```python
from build123d import *

# Parameters (mm, degrees)
F0_R     = 19.05
F0_R_2   = 17.5
F0_R_3   = 9
F1_DEPTH = 88.9
F2_DEPTH = 13
F3_R     = 17.5
F3_R_2   = 9
F4_DEPTH = 13
F6_W     = 19.05
F6_H     = 15.875
F7_DEPTH = 2.54
F8_D     = 3.7973
F8_DEPTH = 12.7
F8_START = 2.54
F8_TIP   = 1.1408240143


with BuildPart() as f1:
    # F0 (on Top) → F1 (new body)
    with BuildSketch(Plane.XY):
        Circle(F0_R)
        Circle(F0_R_2, mode=Mode.SUBTRACT)
        Circle(F0_R_2)
        Circle(F0_R_3, mode=Mode.SUBTRACT)
    extrude(amount=F1_DEPTH)

    # F0 (on Top) → F2 (cut)
    with BuildSketch(Plane.XY):
        Circle(F0_R_2)
        Circle(F0_R_3, mode=Mode.SUBTRACT)
    extrude(amount=F2_DEPTH, mode=Mode.SUBTRACT)

    # F3 (on face) → F4 (cut)
    with BuildSketch(Plane.XY.offset(88.9)):
        Circle(F3_R)
        Circle(F3_R_2, mode=Mode.SUBTRACT)
    extrude(amount=-F4_DEPTH, mode=Mode.SUBTRACT)

    # F6 (on offset) → F7 (cut)
    with BuildSketch(Plane.XZ.offset(19.05)):
        with Locations((0, 63.5)):
            Rectangle(F6_W, F6_H)
    extrude(amount=-F7_DEPTH, mode=Mode.SUBTRACT)

    # F8
    # its depths count from where the whole tool has entered the part; down to there all is cleared
    with Locations(Plane.XZ.offset(19.05).offset(-F8_START)):
        with Locations((0, 63.5)):
            Hole(F8_D / 2, depth=F8_DEPTH)
            with Locations((0, 0, -(F8_DEPTH + F8_TIP / 2))):  # 118° drill point
                Cone(0, F8_D / 2, F8_TIP, mode=Mode.SUBTRACT)


solid = f1.part
```
Input: part model. Units: mm. Frame: model coordinates. A direction names the side the tool comes from. Give positions to 0.01 mm unless a question says otherwise; leave off trailing zeros. Order: outer loops, then holes, each group sorted by start corner. A loop starts at its lowest first (then second) coordinate and runs counter-clockwise, first axis right, second up. Notation, with made-up numbers: (0, 13) -> (8, 13) arc R7 ccw to (8, 24) -> close; hole circle Ø10 at (-24.75, 44.5). An arc over 180 degrees is marked (long way). Write each question's results on one line, items separated by ' | '. Start each with the question number.
Item 1: Cut plane A-A on x = 0. Return the cut outline in (y, z).
Item 2: Cut plane C-C on y = -13. Return the cut outline in (x, z), then the cut area to 3 significant figures.
Item 3: Cut plane D-D on x = -14. Return the cut outline in (y, z), then the cut area to 3 significant figures.
Item 4: Mould query, pull axis Y, two halves, no side actions, for faces 4 (the cylindrical face through (-2.48, 18.888, 43.828)), 5 (the flat face through (17, -6, 0)), 6 (the cylindrical face through (-1.172, 8.923, 44.01)). Classes: pulls with the +Y half, pulls with the -Y half, needs draft (parallel to the pull), parting line crosses it, or undercut.
Item 5: Set-up query: faces 1 (the flat face through (0, -18, 55.562)), 2 (the cylindrical face through (0.412, -12.597, 61.646)), 3 (the flat face through (8, -8, 75.9)). Return all of +Z, -Z, +X, -X, +Y, -Y with unobstructed straight access to the full face (end or side cutting, diameter ignored); none if empty.
Item 6: Contact query for flat-ended pins moving along their axis: P1, Ø3.5, axis at x = 0, z = 63.5, coming from the -Y side; P2, Ø17.5, axis at x = -8, y = -2, coming from the -Z side; P3, Ø6, axis at x = 4.5, y = -1.5, coming from the +Z side; P4, Ø6, axis at x = -14, z = 68.5, coming from the +Y side. Output: stop coordinate, or through.
Item 7: Line query: line 1 (Y direction, x = 0, z = 85.25); line 2 (Y direction, x = 0, z = 36); line 3 (Z direction, x = 0, y = -13.5). Output: solid intervals per line, ascending.
Item 8: Cut plane B-B on y = 0. Return the cut outline in (x, z).
Established:
1) outline: (-19.05, 0) -> (-17.5, 0) -> (-17.5, 13) -> (-9, 13) -> (-9, 61.6) -> (-16.51, 61.6) -> (-16.51, 55.56) -> (-19.05, 55.56) -> close; (-19.05, 71.44) -> (-16.51, 71.44) -> (-16.51, 65.4) -> (-9, 65.4) -> (-9, 75.9) -> (-17.5, 75.9) -> (-17.5, 88.9) -> (-19.05, 88.9) -> close; (9, 13) -> (17.5, 13) -> (17.5, 0) -> (19.05, 0) -> (19.05, 88.9) -> (17.5, 88.9) -> (17.5, 75.9) -> (9, 75.9) -> close
2) outline: (-13.92, 0) -> (-11.72, 0) -> (-11.72, 13) -> (11.72, 13) -> (11.72, 0) -> (13.92, 0) -> (13.92, 88.9) -> (11.72, 88.9) -> (11.72, 75.9) -> (-11.72, 75.9) -> (-11.72, 88.9) -> (-13.92, 88.9) -> close; hole circle Ø3.8 at (0, 63.5) | area: 1,860 mm^2
3) outline: (-12.92, 0) -> (-10.5, 0) -> (-10.5, 13) -> (10.5, 13) -> (10.5, 0) -> (12.92, 0) -> (12.92, 88.9) -> (10.5, 88.9) -> (10.5, 75.9) -> (-10.5, 75.9) -> (-10.5, 88.9) -> (-12.92, 88.9) -> close | area: 1,750 mm^2
4) face 4: parting line crosses it | face 5: needs draft | face 6: undercut
5) face 1: +X, -X, -Y | face 2: -Y | face 3: +Z
6) P1: y = 8.83 | P2: z = 13 | P3: through | P4: y = 15.55
7) line 1: -19.05 to -17.5, 17.5 to 19.05 | line 2: -19.05 to -9, 9 to 19.05 | line 3: 13 to 61.6, 65.4 to 75.9
8) outline: (-19.05, 0) -> (-17.5, 0) -> (-17.5, 13) -> (-9, 13) -> (-9, 75.9) -> (-17.5, 75.9) -> (-17.5, 88.9) -> (-19.05, 88.9) -> close; (9, 13) -> (17.5, 13) -> (17.5, 0) -> (19.05, 0) -> (19.05, 88.9) -> (17.5, 88.9) -> (17.5, 75.9) -> (9, 75.9) -> close
